```python
from build123d import *

# Parameters (mm, degrees)
BOSS_EXTRUDE1_DEPTH     = 54.2
BOSS_EXTRUDE2_DEPTH     = 1.1
SKETCH3_R               = 1.1
CUT_EXTRUDE1_DEPTH      = 31
CUT_EXTRUDE2_DEPTH      = 14.4
SKETCH5_R               = 1.1
CUT_EXTRUDE3_DEPTH      = 31
CUT_EXTRUDE4_DEPTH      = 14.4
CUT_EXTRUDE5_DEPTH      = 6
CUT_EXTRUDE5_DEPTH_BACK = 6
SKETCH7_W               = 34.1
SKETCH7_H               = 0.4
CUT_EXTRUDE6_DEPTH      = 1.9
CUT_EXTRUDE7_DEPTH      = 1.9
SKETCH14_W              = 0.5
SKETCH14_H              = 2.4
BOSS_EXTRUDE3_DEPTH     = 2.5
SKETCH15_W              = 0.5
SKETCH15_H              = 2.4
BOSS_EXTRUDE4_DEPTH     = 2.5
SKETCH16_W              = 0.5
SKETCH16_H              = 2.4
BOSS_EXTRUDE5_DEPTH     = 2.5
SKETCH17_W              = 0.5
SKETCH17_H              = 2.4
BOSS_EXTRUDE6_DEPTH     = 2.5
BOSS_EXTRUDE7_DEPTH     = 4.5
BOSS_EXTRUDE8_DEPTH     = 4.5


with BuildPart() as part:
    # Sketch1 → Boss-Extrude1 (new body)
    with BuildSketch(Plane.XY.offset(-23.2)):
        with BuildLine():
            Line((-5.1, 29.150999964), (-5.1, 0))
            Line((-5.1, 0), (5.1, 0))
            Line((5.1, 0), (5.1, 29.150999964))
            ThreePointArc((5.1, 29.150999964), (5.005777258, 29.443138316), (4.758620732, 29.625172362))
            ThreePointArc((4.758620732, 29.625172362), (2.2e-08, 30.4), (-4.75862069, 29.625172376))
            ThreePointArc((-4.75862069, 29.625172376), (-5.005777245, 29.443138334), (-5.1, 29.150999964))
        make_face()
    extrude(amount=BOSS_EXTRUDE1_DEPTH)

    # Sketch2 → Boss-Extrude2 (add)
    with BuildSketch(Plane(origin=(0, 29.4, 0), x_dir=(1, 0, 0), z_dir=(0, 1, 0))):
        Polygon((-2.09375, 1.5), (-1.40625, 1.5), (-1.40625, 3.25), (-0.59375, 4.0625), (1.21875, 1.5), (2.09375, 1.5), (-0.09375, 4.5625), (1.90625, 6.5), (1.03125, 6.5), (-1.40625, 4.125), (-1.40625, 6.5), (-2.09375, 6.5), align=None)
    extrude(amount=BOSS_EXTRUDE2_DEPTH)

    # Sketch3 → Cut-Extrude1 (cut)
    with BuildSketch(Plane(origin=(0, 30.4, 0), x_dir=(1, 0, 0), z_dir=(0, 1, 0))):
        with Locations(Location((3.2, -20.75, 0), (0, 0, 270))):
            Circle(SKETCH3_R)
    extrude(amount=-CUT_EXTRUDE1_DEPTH, mode=Mode.SUBTRACT)

    # Sketch4 → Cut-Extrude2 (cut)
    with BuildSketch(Plane(origin=(0, 30.4, 0), x_dir=(1, 0, 0), z_dir=(0, 1, 0))):
        with BuildLine():
            Line((3.2, -22.85), (4.7, -22.85))
            ThreePointArc((4.7, -22.85), (4.982842712, -22.967157288), (5.1, -23.25))
            Line((5.1, -23.25), (6.2, -23.25))
            Line((6.2, -23.25), (6.2, -18.25))
            Line((6.2, -18.25), (5.1, -18.25))
            ThreePointArc((5.1, -18.25), (4.982842712, -18.532842712), (4.7, -18.65))
            Line((4.7, -18.65), (3.2, -18.65))
            ThreePointArc((3.2, -18.65), (1.1, -20.75), (3.2, -22.85))
        make_face()
    extrude(amount=-CUT_EXTRUDE2_DEPTH, mode=Mode.SUBTRACT)

    # Sketch5 → Cut-Extrude3 (cut)
    with BuildSketch(Plane(origin=(0, 30.4, 0), x_dir=(1, 0, 0), z_dir=(0, 1, 0))):
        with Locations(Location((-3.2, -28.9, 0), (0, 0, 270))):
            Circle(SKETCH5_R)
    extrude(amount=-CUT_EXTRUDE3_DEPTH, mode=Mode.SUBTRACT)

    # Sketch6 → Cut-Extrude4 (cut)
    with BuildSketch(Plane(origin=(0, 30.4, 0), x_dir=(1, 0, 0), z_dir=(0, 1, 0))):
        with BuildLine():
            Line((-6.2, -26.4), (-6.2, -31.9))
            Line((-6.2, -31.9), (-0.7, -31.9))
            Line((-0.7, -31.9), (-0.7, -31))
            ThreePointArc((-0.7, -31), (-0.982842712, -30.882842712), (-1.1, -30.6))
            Line((-1.1, -30.6), (-1.1, -28.9))
            ThreePointArc((-1.1, -28.9), (-1.71507576, -27.41507576), (-3.2, -26.8))
            Line((-3.2, -26.8), (-4.7, -26.8))
            ThreePointArc((-4.7, -26.8), (-4.982842712, -26.682842712), (-5.1, -26.4))
            Line((-5.1, -26.4), (-6.2, -26.4))
        make_face()
    extrude(amount=-CUT_EXTRUDE4_DEPTH, mode=Mode.SUBTRACT)

    # Sketch7 → Cut-Extrude5 (cut, two sides: drawn at the far end of the back side and taken through both)
    with BuildSketch(Plane(origin=(0, 0, 0), x_dir=(0, 0, -1), z_dir=(1, 0, 0)).offset(-CUT_EXTRUDE5_DEPTH_BACK)):
        with Locations((6.17, 0.2)):
            Rectangle(SKETCH7_W, SKETCH7_H)
    extrude(amount=CUT_EXTRUDE5_DEPTH + CUT_EXTRUDE5_DEPTH_BACK, mode=Mode.SUBTRACT)

    # Sketch8 → Cut-Extrude6 (cut)
    with BuildSketch(Plane(origin=(0, 0, 0), x_dir=(1, 0, 0), z_dir=(0, 1, 0))):
        with BuildLine():
            Line((-3.15, 2.465258607), (-3.15, -2.465258607))
            ThreePointArc((-3.15, -2.465258607), (0, -4), (3.15, -2.465258607))
            Line((3.15, -2.465258607), (3.15, 2.465258607))
            ThreePointArc((3.15, 2.465258607), (0, 4), (-3.15, 2.465258607))
        make_face()
    extrude(amount=CUT_EXTRUDE6_DEPTH, mode=Mode.SUBTRACT)

    # Sketch9 → Cut-Extrude7 (cut)
    with BuildSketch(Plane(origin=(0, 0, 0), x_dir=(1, 0, 0), z_dir=(0, 1, 0))):
        with BuildLine():
            Line((-3.15, 17.165258607), (-3.15, 12.234741393))
            ThreePointArc((-3.15, 12.234741393), (0, 10.7), (3.15, 12.234741393))
            Line((3.15, 12.234741393), (3.15, 17.165258607))
            ThreePointArc((3.15, 17.165258607), (0, 18.7), (-3.15, 17.165258607))
        make_face()
    extrude(amount=CUT_EXTRUDE7_DEPTH, mode=Mode.SUBTRACT)

    # Sketch10 → Revolve1 (revolve)
    with BuildSketch(Plane(origin=(0, 0, 0), x_dir=(0, 0, -1), z_dir=(1, 0, 0)), mode=Mode.PRIVATE) as revolve1_sk:
        Polygon((0, 2.1), (3.05, 2.1), (3.05, 1.1), (2.25, 1.1), (2.25, -1.4), (2.65, -1.4), (2.65, -1.72), (2.430606898, -2.1), (0, -2.1), align=None)
    revolve(revolve1_sk.sketch.rotate(Axis((0, -2.1, 0), (0, 1, 0)), 180), axis=Axis((0, -2.1, 0), (0, 1, 0)))

    # Sketch11 → Revolve2 (revolve)
    with BuildSketch(Plane(origin=(0, 0, 0), x_dir=(0, 0, -1), z_dir=(1, 0, 0)), mode=Mode.PRIVATE) as revolve2_sk:
        Polygon((14.7, 2.1), (17.75, 2.1), (17.75, 1.1), (16.95, 1.1), (16.95, -1.4), (17.35, -1.4), (17.35, -1.72), (17.130606898, -2.1), (14.7, -2.1), align=None)
    revolve(revolve2_sk.sketch.rotate(Axis((0, -2.1, -14.7), (0, 1, 0)), 180), axis=Axis((0, -2.1, -14.7), (0, 1, 0)))

    # Sketch12 → Revolve3 (revolve)
    with BuildSketch(Plane.XY.offset(-7.35), mode=Mode.PRIVATE) as revolve3_sk:
        with BuildLine():
            Line((2.6, 0.4), (3.8, 0.4))
            Line((3.8, 0.4), (3.6, -6.9))
            ThreePointArc((3.6, -6.9), (3.106540729, -7.021444616), (2.6, -7.06227766))
            Line((2.6, -7.06227766), (2.6, 0.4))
        make_face()
    revolve(revolve3_sk.sketch.rotate(Axis((2.6, -7.06227766, -7.35), (0, 1, 0)), 270), axis=Axis((2.6, -7.06227766, -7.35), (0, 1, 0)))

    # Sketch13 → Revolve4 (revolve)
    with BuildSketch(Plane.XY.offset(-7.35), mode=Mode.PRIVATE) as revolve4_sk:
        with BuildLine():
            Line((-2.6, 0.4), (-1.4, 0.4))
            Line((-1.4, 0.4), (-1.6, -6.9))
            ThreePointArc((-1.6, -6.9), (-2.093459271, -7.021444616), (-2.6, -7.06227766))
            Line((-2.6, -7.06227766), (-2.6, 0.4))
        make_face()
    revolve(revolve4_sk.sketch.rotate(Axis((-2.6, -7.06227766, -7.35), (0, 1, 0)), 270), axis=Axis((-2.6, -7.06227766, -7.35), (0, 1, 0)))

    # Sketch14 → Boss-Extrude3 (add)
    with BuildSketch(Plane(origin=(0, -2.1, 0), x_dir=(-1, 0, 0), z_dir=(0, -1, 0))):
        with Locations((-1, 0)):
            Rectangle(SKETCH14_W, SKETCH14_H)
    extrude(amount=BOSS_EXTRUDE3_DEPTH)

    # Sketch15 → Boss-Extrude4 (add)
    with BuildSketch(Plane(origin=(0, -2.1, 0), x_dir=(-1, 0, 0), z_dir=(0, -1, 0))):
        with Locations((1, 0)):
            Rectangle(SKETCH15_W, SKETCH15_H)
    extrude(amount=BOSS_EXTRUDE4_DEPTH)

    # Sketch16 → Boss-Extrude5 (add)
    with BuildSketch(Plane(origin=(0, -2.1, 0), x_dir=(-1, 0, 0), z_dir=(0, -1, 0))):
        with Locations((-1, 14.7)):
            Rectangle(SKETCH16_W, SKETCH16_H)
    extrude(amount=BOSS_EXTRUDE5_DEPTH)

    # Sketch17 → Boss-Extrude6 (add)
    with BuildSketch(Plane(origin=(0, -2.1, 0), x_dir=(-1, 0, 0), z_dir=(0, -1, 0))):
        with Locations((1, 14.7)):
            Rectangle(SKETCH17_W, SKETCH17_H)
    extrude(amount=BOSS_EXTRUDE6_DEPTH)

    # Sketch18 → Revolve5 (revolve)
    with BuildSketch(Plane(origin=(0, 0, 0), x_dir=(0, 0, -1), z_dir=(1, 0, 0)), mode=Mode.PRIVATE) as revolve5_sk:
        with BuildLine():
            Line((-3.2, 32.4), (-2.75, 32.4))
            Line((-2.75, 32.4), (-2.35, 32.8))
            Line((-2.35, 32.8), (-1.9, 32.8))
            Line((-1.9, 32.8), (-1.9, 31.943560486))
            ThreePointArc((-1.9, 31.943560486), (-0.666287758, 31.784461515), (0.549999769, 31.523687608))
            ThreePointArc((0.549999769, 31.523687608), (0.766227693, 31.381338282), (0.85, 31.136389214))
            Line((0.85, 31.136389214), (0.85, 28.1))
            Line((0.85, 28.1), (-3.2, 28.1))
            Line((-3.2, 28.1), (-3.2, 32.4))
        make_face()
    revolve(revolve5_sk.sketch.rotate(Axis((0, 28.1, 3.2), (0, 1, 0)), 180), axis=Axis((0, 28.1, 3.2), (0, 1, 0)))

    # Sketch19 → Revolve6 (revolve)
    with BuildSketch(Plane(origin=(0, 0, 0), x_dir=(0, 0, -1), z_dir=(1, 0, 0)), mode=Mode.PRIVATE) as revolve6_sk:
        with BuildLine():
            Line((11.5, 32.4), (11.95, 32.4))
            Line((11.95, 32.4), (12.35, 32.8))
            Line((12.35, 32.8), (12.8, 32.8))
            Line((12.8, 32.8), (12.8, 31.943560486))
            ThreePointArc((12.8, 31.943560486), (14.033712242, 31.784461515), (15.249999769, 31.523687608))
            ThreePointArc((15.249999769, 31.523687608), (15.466227693, 31.381338282), (15.55, 31.136389214))
            Line((15.55, 31.136389214), (15.55, 28.1))
            Line((15.55, 28.1), (11.5, 28.1))
            Line((11.5, 28.1), (11.5, 32.4))
        make_face()
    revolve(revolve6_sk.sketch.rotate(Axis((0, 28.1, -11.5), (0, 1, 0)), 180), axis=Axis((0, 28.1, -11.5), (0, 1, 0)))

    # Sketch20 → Cut-Revolve1 (revolve, cut)
    with BuildSketch(Plane.XY.offset(26.6), mode=Mode.PRIVATE) as cut_revolve1_sk:
        Polygon((1.75, 30.5), (2.25, 30.5), (2.25, 25.3), (1.75, 25.011324865), align=None)
    revolve(cut_revolve1_sk.sketch.rotate(Axis((1.75, 25.011324865, 26.6), (0, 1, 0)), 270), axis=Axis((1.75, 25.011324865, 26.6), (0, 1, 0)), mode=Mode.SUBTRACT)

    # Sketch21 → Boss-Extrude7 (add)
    with BuildSketch(Plane.XY.offset(-23.3)):
        with BuildLine():
            Line((0.75, 30.481362671), (0.75, 27))
            Line((0.75, 27), (2.75, 27))
            Line((2.75, 27), (2.75, 30.247474533))
            ThreePointArc((2.75, 30.247474533), (1.753903052, 30.397793974), (0.75, 30.481362671))
        make_face()
    extrude(amount=BOSS_EXTRUDE7_DEPTH)

    # Sketch22 → Boss-Extrude8 (add)
    with BuildSketch(Plane.XY.offset(-23.3)):
        with BuildLine():
            Line((-2.75, 30.247474533), (-2.75, 27))
            Line((-2.75, 27), (-0.75, 27))
            Line((-0.75, 27), (-0.75, 30.481362671))
            ThreePointArc((-0.75, 30.481362671), (-1.753903052, 30.397793974), (-2.75, 30.247474533))
        make_face()
    extrude(amount=BOSS_EXTRUDE8_DEPTH)


solid = part.part
```
Build history of the part. All positions in model axes, mm. A direction names the side the tool comes from. Coordinates: 2 decimals unless noted, no trailing zeros. Order: outer loops, then holes, each group sorted by start corner. A loop starts at its lowest first (then second) coordinate and runs counter-clockwise, first axis right, second up.
Item 1: Saw through at A-A on y = 3. List the corners of the cut face in (x, z).
Filled in:
outline: (-5.1, -23.2) - (5.1, -23.2) - (5.1, 31) - (-5.1, 31) - close; hole circle Ø2.2 at (-3.2, 28.9); hole circle Ø2.2 at (3.2, 20.75)
Item 2: Tool access for faces 1 (the cylindrical face through (-1.74, 30.4, -21.08)), 2 (the flat face through (0.75, -3, -15)), 3 (the flat face through (-3.15, 0.97, -0.03)), 4 (the flat face through (4, 23, 22.85)): list every direction of +Z, -Z, +X, -X, +Y, -Y with a clear straight run to the whole face (end or side of a thin tool).
Filled in:
face 1: -Z, -X, +Y
face 2: +Z, -Z, -Y
face 3: -Y
face 4: +X, +Y
Item 3: Drill centre lines: L1, parallel to Z at x = 1.75, y = 29.05; L2, parallel to Y at x = 2, z = -16; L3, parallel to Y at x = -1.5, z = 13. Where is each one in solid material? Low to high.
Filled in:
L1: z = -23.3 to 19.23, 22.27 to 26.1, 27.1 to 31
L2: y = -2.1 to -1.4, 1.1 to 30.27
L3: y = 0 to 30.32
Item 4: Mould opens along X. For faces 5 (the flat face through (2, 29, -23.3)), 6 (the flat face through (0, -2.1, -15)), 7 (the cylindrical face through (3.4, 30.6, -9.3)) say: released by +X, released by -X, zero draft, split by the parting line, or undercut.
Filled in:
face 5: zero draft
face 6: undercut
face 7: split by the parting line
Item 5: Drop flat-ended pins along their axis: pin 1 Ø1.2 at (y, z) = (-3, -14.5) entering from +X; pin 2 Ø2 at (x, y) = (3, -1) entering from -Z; pin 3 Ø3 at (x, z) = (-1, -6.5) entering from -Y. Give the stop position or say it passes through.
Filled in:
pin 1: stops at x = 1.25
pin 2: stops at z = -16.34
pin 3: stops at y = -7.05
